Model file for the job. Use its own axes, mm. Give positions to 0.01 mm unless a question says otherwise; leave off trailing zeros. Write each loop counter-clockwise with the first axis right and the second up, starting at its lowest first coordinate (ties: lowest second). Pieces come first, ordered by that corner, then holes.
```python
from build123d import *

# Parameters (mm, degrees)
SKETCH1_R                = 30.48
BOSS_EXTRUDE1_DEPTH      = 25.4
F_1_4_28_TAPPED_HOLE1_D  = 5.4102
F_1_4_CLEARANCE_HOLE2_D  = 6.5278
CUT_EXTRUDE1_DEPTH       = 51.032197633
FILLET1_R                = 2.54
CIRPATTERN1_COUNT        = 6
FILLET1_OF_CIRPATTERN1_R = 2.54
SKETCH8_R                = 20.6502
CUT_EXTRUDE2_DEPTH       = 6.35


with BuildPart() as part:
    # Sketch1 → Boss-Extrude1 (new body)
    with BuildSketch(Plane(origin=(0, 0, 0), x_dir=(1, 0, 0), z_dir=(0, 1, 0))):
        with Locations(Location((0, 0, 0), (0, 0, 270))):
            Circle(SKETCH1_R)
    extrude(amount=BOSS_EXTRUDE1_DEPTH)

    # 1/4-28 Tapped Hole1 (through all)
    with Locations(Plane(origin=(0, 25.4, 0), x_dir=(1, 0, 0), z_dir=(0, 1, 0))):
        with Locations((0, 0)):
            Hole(F_1_4_28_TAPPED_HOLE1_D / 2)

    # 1/4 Clearance Hole2 (through all)
    with Locations(Plane(origin=(0, 0, 0), x_dir=(-1, 0, 0), z_dir=(0, -1, 0))):
        with Locations((269.174368783, -128.772908827), (-18.058184892, -18.021920393), (6.578348439, -24.649807059), (-24.636533331, 6.627886666), (-6.578348439, 24.649807059), (18.058184892, 18.021920393), (24.636533331, -6.627886666)):
            Hole(F_1_4_CLEARANCE_HOLE2_D / 2)

    # Sketch7 → Cut-Extrude1 (cut, through all)
    with BuildSketch(Plane(origin=(0, 25.4, 0), x_dir=(1, 0, 0), z_dir=(0, 1, 0))):
        with BuildLine():
            Line((-13.451907307, 15.667704039), (-0.82483254, 3.065987))
            Line((-0.82483254, 3.065987), (3.775037164, 20.302213043))
            ThreePointArc((3.775037164, 20.302213043), (-5.364710837, 19.941179445), (-13.451907307, 15.667704039))
        make_face()
    cut_extrude1 = extrude(amount=-CUT_EXTRUDE1_DEPTH, mode=Mode.SUBTRACT)

    # Fillet1
    fillet1_edges = [part.edges().sort_by_distance(p)[0] for p in [
        (-13.451907307, 12.7, -15.667704039),
        (3.775037164, 12.7, -20.302213043),
        (-0.82483254, 12.7, -3.065987),
    ]]
    fillet(fillet1_edges, radius=FILLET1_R)

    # CirPattern1: Cut-Extrude1 ×6 about axis
    cirpattern1_axis = Axis((0, 0, 0), (0, 1, 0))
    for i in range(1, CIRPATTERN1_COUNT):
        add(cut_extrude1.rotate(cirpattern1_axis, i * 360 / CIRPATTERN1_COUNT), mode=Mode.SUBTRACT)

    # Fillet1 of CirPattern1
    fillet1_of_cirpattern1_edges = [part.edges().sort_by_distance(p)[0] for p in [
        (-20.29458337, 12.7, 3.815841438),
        (-15.694713666, 12.7, -13.420384606),
        (-3.067638899, 12.7, -0.818667567),
        (-6.842676063, 12.7, 19.483545477),
        (-19.46975083, 12.7, 6.881828437),
        (-2.24280636, 12.7, 2.247319433),
        (13.451907307, 12.7, 15.667704039),
        (-3.775037164, 12.7, 20.302213043),
        (0.82483254, 12.7, 3.065987),
        (20.29458337, 12.7, -3.815841438),
        (15.694713666, 12.7, 13.420384606),
        (3.067638899, 12.7, 0.818667567),
        (6.842676063, 12.7, -19.483545477),
        (19.46975083, 12.7, -6.881828437),
        (2.24280636, 12.7, -2.247319433),
    ]]
    fillet(fillet1_of_cirpattern1_edges, radius=FILLET1_OF_CIRPATTERN1_R)

    # Sketch8 → Cut-Extrude2 (cut)
    with BuildSketch(Plane.XZ.offset(-25.4)):
        with Locations(Location((0, 0, 0), (0, 0, 90))):
            Circle(SKETCH8_R)
    extrude(amount=CUT_EXTRUDE2_DEPTH, mode=Mode.SUBTRACT)


solid = part.part
```
1. Pull direction X, two halves, no side cores. Call faces 1 (the flat face through (-9.84, 9.66, -7.58)), 2 (the flat face through (-20, 25.4, 6)): +X half, -X half, draft (parallel to the pull), parting line (faces both ways), or undercut.
Calculated:
face 1: undercut
face 2: draft
2. Probe probe 1 along Z at (x, y) = (8.5, 16.5); probe 2 along X at (y, z) = (11.25, -14.5); probe 3 along Z at (x, y) = (18, 20.25). List the from-to ranges inside material, lowest first.
Calculated:
probe 1: z = -29.27 to -27.29, -22.01 to -18.51, -3.93 to -0.64, 6.24 to 10.73, 18.82 to 29.27
probe 2: x = -26.81 to -11.95, 2.23 to 5.51, 14.7 to 26.81
probe 3: z = -24.6 to -10.12, 10.12 to 14.76, 21.29 to 24.6
3. Slice it at B-B, the plane y = 21.25. Write the cut outline in (x, z).
Calculated:
outline: circle Ø60.96 at (0, 0); hole circle Ø6.53 at (-24.64, 6.63); hole circle Ø6.53 at (-18.06, -18.02); hole circle Ø41.3 at (0, 0); hole circle Ø6.53 at (-6.58, 24.65); hole circle Ø6.53 at (6.58, -24.65); hole circle Ø6.53 at (18.06, 18.02); hole circle Ø6.53 at (24.64, -6.63)
4. Slice it at A-A, the plane x = 24. Write the cut outline in (y, z), and give its area (3 significant figures).
Calculated:
outline: (0, -18.79) - (25.4, -18.79) - (25.4, -9.83) - (0, -9.83) - close; (0, -3.43) - (25.4, -3.43) - (25.4, 18.79) - (0, 18.79) - close
area: 792 mm2
5. Slice it at C-C, the plane y = 3.5. State how many separate pieces and enclosed holes the cut face has, and give its area (3 significant figures).
Calculated:
separate pieces: 1
enclosed holes: 13
area: 1,770 mm2
6. Pin check, flat tips, straight feed: P1, Ø3, axis at y = 16.5, z = 10.5, coming from the -X side; P2, Ø1.5, axis at y = 13, z = -10, coming from the +X side; P3, Ø6, axis at y = 12, z = 0, coming from the -X side. Stop position of each tip, or through.
Calculated:
P1: stops at x = -29.12
P2: stops at x = 29.04
P3: stops at x = -30.48
